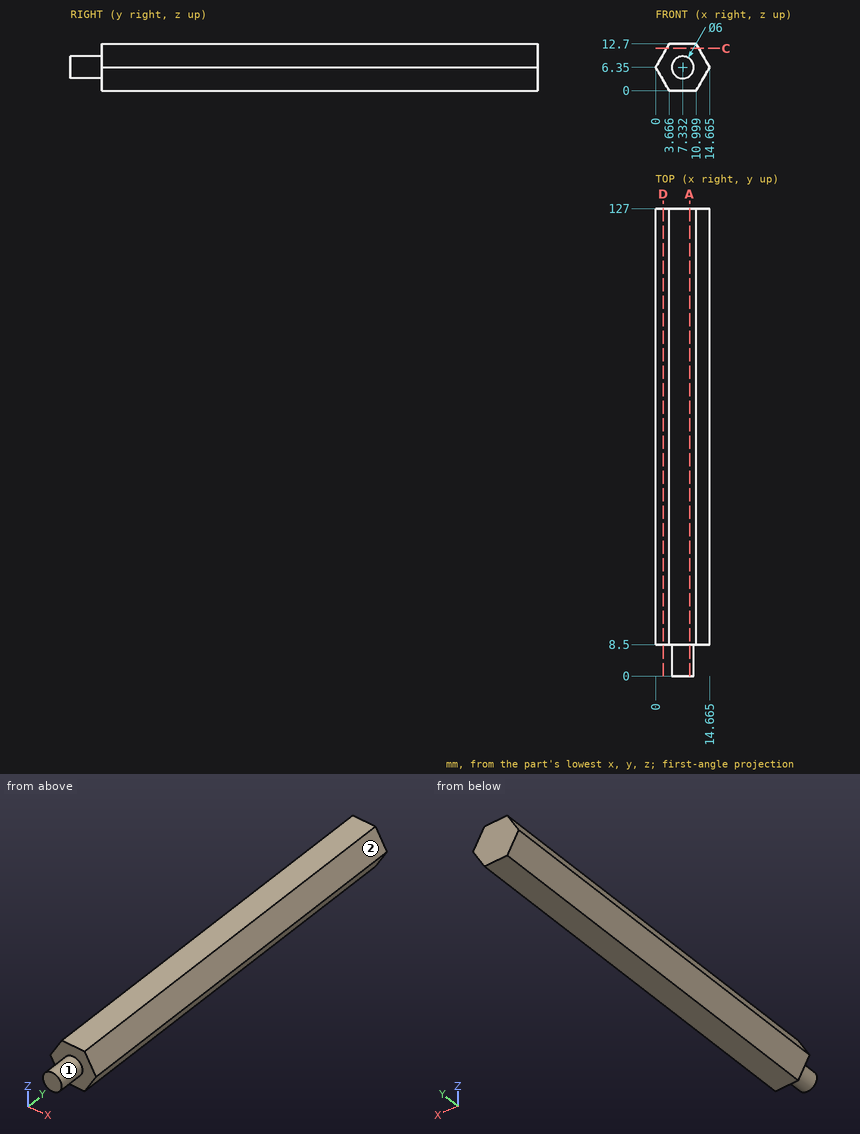
Here's the drawing with two shaded views (mm, measured from the low corner). I have some questions. A direction names the side the tool comes from. Give positions to 0.01 mm unless a question says otherwise; leave off trailing zeros. Order: outer loops, then holes, each group sorted by start corner. A loop starts at its lowest first (then second) coordinate and runs counter-clockwise, first axis right, second up. Notation, with made-up numbers: (66, 57.25) -> (79, 57.25) arc R23 ccw to (79, 82.25) -> close; hole circle Ø5 at (77, 66.5). An arc over 180 degrees is marked (long way). One line per item, written item: value. Start each with the question number.
1. Will these pins go through, and if not, where does the flat tip stop? pin 1 Ø5 at (y, z) = (55, 5.5) entering from -X; pin 2 Ø3 at (y, z) = (13.5, 8) entering from +X.
2. For the marked faces 1 and 2, which set-ups out of +Z, -Z, +X, -X, +Y, -Y let a thin tool reach every point of the face, with its end or its side?
3. I need wall thicknesses on probe 1 along Y at (x, z) = (10.25, 3.75); probe 2 along X at (y, z) = (116.5, 5.5) (1 decimal); probe 3 along X at (y, z) = (39, 5.25) (1 decimal). Which ranges of each line are inside material? Lowest first, please. Write a range as from..to.
4. Imagine slicing it at C-C, the plane z = 11.5. List the corners of the cut face in (x, y) for me, plus the area to 3 significant figures.
5. Imagine slicing it at D-D, the plane x = 2. List the corners of the cut face in (y, z) for me (1 decimal), plus the area to 3 significant figures.
6. Imagine slicing it at A-A, the plane x = 9.25. List the corners of the cut face in (y, z) for me, plus the area to 3 significant figures.
Values follow:
1. pin 1: stops at x = 0
1. pin 2: stops at x = 14.58
2. face 1: -Y
2. face 2: +Z, +X, +Y, -Y
3. probe 1: y = 8.5..127
3. probe 2: x = 0.5..14.2
3. probe 3: x = 0.6..14
4. outline: (2.97, 8.5) -> (11.69, 8.5) -> (11.69, 127) -> (2.97, 127) -> close
4. area: 1,030 mm2
5. outline: (8.5, 2.9) -> (127, 2.9) -> (127, 9.8) -> (8.5, 9.8) -> close
5. area: 821 mm2
6. outline: (0, 4.04) -> (8.5, 4.04) -> (8.5, 0) -> (127, 0) -> (127, 12.7) -> (8.5, 12.7) -> (8.5, 8.66) -> (0, 8.66) -> close
6. area: 1,540 mm2
